Source: CAD feature listing. Evaluate the final solid. Frame: model axes, mm. A direction names the side the tool comes from. Coordinates: 2 decimals unless noted, no trailing zeros. Order: outer loops, then holes, each group sorted by start corner. A loop starts at its lowest first (then second) coordinate and runs counter-clockwise, first axis right, second up.
```python
from build123d import *

# Parameters (mm, degrees)
SKETCH2_R                  = 6.35
BOSS_EXTRUDE1_DEPTH        = 3.175
F_1_4_CLEARANCE_HOLE1_D    = 6.5278
F_10_32_TAPPED_HOLE1_D     = 4.0386
F_10_32_TAPPED_HOLE1_DEPTH = 12.7
F_10_32_TAPPED_HOLE1_TIP   = 1.213317848


with BuildPart() as part:
    # Sketch2 → Boss-Extrude1 (new, symmetric)
    with BuildSketch(Plane(origin=(0, 0, 0), x_dir=(0, 0, -1), z_dir=(1, 0, 0))):
        with BuildLine():
            Line((-50.8, 0), (50.8, 0))
            Line((50.8, 0), (50.8, -82.55))
            ThreePointArc((50.8, -82.55), (0, -133.35), (-50.8, -82.55))
            Line((-50.8, -82.55), (-50.8, 0))
        make_face()
        with Locations((0, -82.55)):
            Circle(SKETCH2_R, mode=Mode.SUBTRACT)
    extrude(amount=BOSS_EXTRUDE1_DEPTH, both=True)

    # 1/4 Clearance Hole1 (through all)
    with Locations(Plane(origin=(3.175, 0, 0), x_dir=(0, 0, -1), z_dir=(1, 0, 0))):
        with Locations((-31.56136055, -64.32803999), (31.56136055, -64.32803999), (0, -118.993920019)):
            Hole(F_1_4_CLEARANCE_HOLE1_D / 2)

    # #10-32 Tapped Hole1
    with Locations(Plane(origin=(0, 0, 0), x_dir=(1, 0, 0), z_dir=(0, 1, 0))):
        with Locations((0, 30.48), (0, 10.16), (0, -10.16), (0, -30.48)):
            Hole(F_10_32_TAPPED_HOLE1_D / 2, depth=F_10_32_TAPPED_HOLE1_DEPTH)
            with Locations((0, 0, -(F_10_32_TAPPED_HOLE1_DEPTH + F_10_32_TAPPED_HOLE1_TIP / 2))):  # 118° drill point
                Cone(0, F_10_32_TAPPED_HOLE1_D / 2, F_10_32_TAPPED_HOLE1_TIP, mode=Mode.SUBTRACT)


solid = part.part
```
1. Section query A-A on y = -8.5. Return loops of the section in (x, z) (3 decimals).
Findings:
outline: (-3.175, -50.8) - (3.175, -50.8) - (3.175, 50.8) - (-3.175, 50.8) - close; hole circle Ø4.039 at (0, -30.48); hole circle Ø4.039 at (0, -10.16); hole circle Ø4.039 at (0, 10.16); hole circle Ø4.039 at (0, 30.48)
2. Access query for faces 1 (the face through (-0.04, -122.18, -0.71)), 2 (the face through (0.4, -6.4, -28.5)). Directions: +Z, -Z, +X, -X, +Y, -Y. A direction counts if a zero-diameter tool reaches every point of the face in a straight line with its end or side. Return the directions, or none.
Findings:
face 1: +X, -X
face 2: +Y
3. Section query D-D on z = 40.5. Return loops of the section in (x, y) (3 decimals), plus the area to 3 significant figures.
Findings:
outline: (-3.175, -113.216) - (3.175, -113.216) - (3.175, 0) - (-3.175, 0) - close
area: 719 mm2
4. Pin query (flat end, axial travel): P1, Ø3.5, axis at x = 0, z = 10.16, coming from the +Y side; P2, Ø2, axis at x = 0.5, y = -104, coming from the -Z side; P3, Ø3, axis at x = 1.5, y = -96.5, coming from the -Z side. Return the tip coordinate at first contact, or that it passes through.
Findings:
P1: stops at y = -12.86
P2: stops at z = -46.5
P3: stops at z = -49.25
5. Section query B-B on y = -87.5. Return loops of the section in (x, z) (3 decimals), plus the area to 3 significant figures.
Findings:
outline: (-3.175, -50.558) - (3.175, -50.558) - (3.175, -3.977) - (-3.175, -3.977) - close; (-3.175, 3.977) - (3.175, 3.977) - (3.175, 50.558) - (-3.175, 50.558) - close
area: 592 mm2
6. Section query C-C on x = -1. Count the separate pieces of the cut face and the enclosed holes in it, plus the area to 3 significant figures.
Findings:
separate pieces: 1
enclosed holes: 4
area: 12,000 mm2
7. Draft query along Y for faces 3 (the face through (-0.076, -13.703, -9.818)), 4 (the face through (-0.044, -61.092, -31.986)), 5 (the face through (0, -41, -50.8)). Return one class per face: released by +Y, released by -Y, zero draft, split by the parting line, or undercut.
Findings:
face 3: released by +Y
face 4: undercut
face 5: zero draft
8. Ray query, line 1 (Z direction, x = 0, y = -10); line 2 (X direction, y = -7, z = 10) (3 decimals); line 3 (Z direction, x = -2.5, y = -78). Return the intervals inside material, ascending.
Findings:
line 1: z = -50.8 to -32.5, -28.46 to -12.18, -8.14 to 8.14, 12.18 to 28.46, 32.5 to 50.8
line 2: x = -3.175 to -2.013, 2.013 to 3.175
line 3: z = -50.8 to -4.43, 4.43 to 50.8
